Here's how the part is built. I have some questions about the finished solid (model axes, mm). Give positions to 0.01 mm unless a question says otherwise; leave off trailing zeros. Order: outer loops, then holes, each group sorted by start corner. A loop starts at its lowest first (then second) coordinate and runs counter-clockwise, first axis right, second up. Notation, with made-up numbers: M -11.5,68.5 L 44.5,68.5 A27 ccw 44.5,94.5 Z; hole C -22,63.25 d7. An arc over 180 degrees is marked long. One line per item, written item: value. Start each with the question number.
from build123d import *

# Parameters (mm, degrees)
BOSS_EXTRUDE1_DEPTH   = 1
SKETCH8_3_R           = 3
CUT_EXTRUDE1_DEPTH    = 182.285837692
CUT_EXTRUDE2_DEPTH    = 182.285837692
SKETCH10_W            = 14.1
SKETCH10_H            = 14.1
CUT_EXTRUDE3_DEPTH    = 185.637780297
F_3_0MM_DOWEL_HOLE1_D = 3
FILLET1_R             = 1


with BuildPart() as part:
    # Sketch8 → Boss-Extrude1 (new body)
    with BuildSketch(Plane.XY):
        with BuildLine():
            ThreePointArc((116.356165737, 89.593531525), (107.510169126, 99.635128091), (106.844308874, 113.000828513))
            ThreePointArc((106.844308874, 113.000828513), (98.551785503, 130.943955248), (79.67265081, 125.087333856))
            ThreePointArc((79.67265081, 125.087333856), (66.957923375, 111.551078569), (49.923987164, 104.152462611))
            ThreePointArc((49.923987164, 104.152462611), (38.279791522, 92.371702096), (44.581782069, 77.053134095))
            ThreePointArc((44.581782069, 77.053134095), (58.651333394, 69.17496271), (73.852303576, 63.794594289))
            ThreePointArc((73.852303576, 63.794594289), (73.863549821, 63.839319131), (73.875482243, 63.883865813))
            ThreePointArc((73.875482243, 63.883865813), (76.767270103, 63.085390407), (79.729789892, 62.612657392))
            ThreePointArc((79.729789892, 62.612657392), (79.717062502, 62.538833177), (79.702495752, 62.465349771))
            ThreePointArc((79.702495752, 62.465349771), (95.373691885, 60.7573177), (111.111302129, 61.669121188))
            ThreePointArc((111.111302129, 61.669121188), (123.74416397, 73.75113123), (116.356165737, 89.593531525))
        make_face()
        with BuildLine():
            ThreePointArc((109.375963817, 92.019534234), (109.377797318, 92.017499849), (109.379631064, 92.015465685))
            ThreePointArc((109.379631064, 92.015465685), (109.377986421, 92.015505684), (109.376341775, 92.015545509))
            ThreePointArc((109.376341775, 92.015545509), (109.37615287, 92.017539878), (109.375963817, 92.019534234))
        make_face(mode=Mode.SUBTRACT)
        with BuildLine():
            ThreePointArc((56.72077423, 104.000844147), (56.721683918, 104.00117089), (56.7225936, 104.001497652))
            ThreePointArc((56.7225936, 104.001497652), (56.755397532, 103.992206145), (56.788325126, 103.983362865))
            ThreePointArc((56.788325126, 103.983362865), (56.754559843, 103.992142785), (56.72077423, 104.000844147))
        make_face(mode=Mode.SUBTRACT)
        with BuildLine():
            ThreePointArc((103.532400156, 106.396636288), (103.543227812, 106.407709628), (103.554044399, 106.418793781))
            ThreePointArc((103.554044399, 106.418793781), (103.552293137, 106.396310438), (103.550744757, 106.373812212))
            ThreePointArc((103.550744757, 106.373812212), (103.541575551, 106.385226737), (103.532400156, 106.396636288))
        make_face(mode=Mode.SUBTRACT)
        with BuildLine():
            ThreePointArc((104.104138674, 107.788453533), (104.062244422, 107.735361058), (104.021801646, 107.681154775))
            ThreePointArc((104.021801646, 107.681154775), (104.021865069, 107.684582448), (104.021929019, 107.688010111))
            ThreePointArc((104.021929019, 107.688010111), (104.063142491, 107.7381429), (104.104138674, 107.788453533))
        make_face(mode=Mode.SUBTRACT)
    extrude(amount=BOSS_EXTRUDE1_DEPTH)

    # Sketch8_3 → Cut-Extrude1 (cut, through all)
    with BuildSketch(Plane.XY):
        with Locations((106.04559389, 106.21341333)):
            Circle(SKETCH8_3_R)
        with Locations((76.767270103, 63.085390407)):
            Circle(SKETCH8_3_R)
        with Locations((57.420286528, 106.402169345)):
            Circle(SKETCH8_3_R)
    extrude(amount=CUT_EXTRUDE1_DEPTH, mode=Mode.SUBTRACT)

    # Sketch14 → Cut-Extrude2 (cut, through all)
    with BuildSketch(Plane.XY):
        with BuildLine():
            Line((54.297852906, 82.909160119), (55.387130976, 81.231818983))
            ThreePointArc((55.387130976, 81.231818983), (54.003821373, 81.525850516), (54.297852906, 82.909160119))
        make_face()
        with BuildLine():
            Line((56.641344681, 93.934422083), (58.318685817, 95.023700153))
            ThreePointArc((58.318685817, 95.023700153), (56.935376214, 95.317731686), (56.641344681, 93.934422083))
        make_face()
        with BuildLine():
            Line((69.343947781, 92.680208378), (70.433225851, 91.002867242))
            ThreePointArc((70.433225851, 91.002867242), (70.727257384, 92.386176845), (69.343947781, 92.680208378))
        make_face()
        with BuildLine():
            Line((68.089734077, 79.977605278), (66.412392941, 78.888327208))
            ThreePointArc((66.412392941, 78.888327208), (67.795702544, 78.594295675), (68.089734077, 79.977605278))
        make_face()
        with BuildLine():
            Line((75.275056475, 89.973704373), (76.952397611, 91.062982443))
            ThreePointArc((76.952397611, 91.062982443), (75.569088008, 91.357013976), (75.275056475, 89.973704373))
        make_face()
        with BuildLine():
            Line((72.9315647, 78.948442409), (74.02084277, 77.271101273))
            ThreePointArc((74.02084277, 77.271101273), (72.637533167, 77.565132806), (72.9315647, 78.948442409))
        make_face()
        with BuildLine():
            Line((85.046104735, 74.927609498), (86.723445871, 76.016887568))
            ThreePointArc((86.723445871, 76.016887568), (86.429414338, 74.633577965), (85.046104735, 74.927609498))
        make_face()
        with BuildLine():
            Line((89.066937645, 87.042149532), (87.977659575, 88.719490668))
            ThreePointArc((87.977659575, 88.719490668), (89.360969178, 88.425459135), (89.066937645, 87.042149532))
        make_face()
        with BuildLine():
            Line((89.006822445, 93.561321292), (90.684163581, 94.650599362))
            ThreePointArc((90.684163581, 94.650599362), (90.390132048, 93.267289759), (89.006822445, 93.561321292))
        make_face()
        with BuildLine():
            Line((76.89228241, 97.582154203), (77.981560481, 95.904813067))
            ThreePointArc((77.981560481, 95.904813067), (76.598250878, 96.1988446), (76.89228241, 97.582154203))
        make_face()
        with BuildLine():
            Line((91.938377285, 107.353202462), (93.027655356, 105.675861326))
            ThreePointArc((93.027655356, 105.675861326), (93.321686888, 107.059170929), (91.938377285, 107.353202462))
        make_face()
        with BuildLine():
            Line((79.235774185, 108.607416167), (80.913115321, 109.696694237))
            ThreePointArc((80.913115321, 109.696694237), (79.529805718, 109.99072577), (79.235774185, 108.607416167))
        make_face()
        with BuildLine():
            Line((93.908768269, 86.012986663), (95.586109405, 87.102264733))
            ThreePointArc((95.586109405, 87.102264733), (94.202799802, 87.396296266), (93.908768269, 86.012986663))
        make_face()
        with BuildLine():
            Line((91.565276494, 74.987724698), (92.654554564, 73.310383563))
            ThreePointArc((92.654554564, 73.310383563), (91.271244961, 73.604415095), (91.565276494, 74.987724698))
        make_face()
        with BuildLine():
            Line((103.679816529, 70.966891788), (105.357157665, 72.056169858))
            ThreePointArc((105.357157665, 72.056169858), (105.063126132, 70.672860255), (103.679816529, 70.966891788))
        make_face()
        with BuildLine():
            Line((106.611371369, 84.758772958), (107.700649439, 83.081431822))
            ThreePointArc((107.700649439, 83.081431822), (107.994680972, 84.464741425), (106.611371369, 84.758772958))
        make_face()
    extrude(amount=CUT_EXTRUDE2_DEPTH, mode=Mode.SUBTRACT)

    # Sketch10 → Cut-Extrude3 (cut, through all)
    with BuildSketch(Plane(origin=(-22.098060608, 19.345391025, 0), x_dir=(0.9781476007338056, -0.2079116908177598, 0), z_dir=(0, 0, 1))):
        with Locations((68.560828803, 83.69413822)):
            Rectangle(SKETCH10_W, SKETCH10_H)
        with Locations((87.610828803, 83.69413822)):
            Rectangle(SKETCH10_W, SKETCH10_H)
        with Locations((106.660828803, 83.69413822)):
            Rectangle(SKETCH10_W, SKETCH10_H)
        with Locations((87.610828803, 102.74413822)):
            Rectangle(SKETCH10_W, SKETCH10_H)
    extrude(amount=CUT_EXTRUDE3_DEPTH, mode=Mode.SUBTRACT)

    # 3.0mm Dowel Hole1 (through all)
    with Locations(Plane.XY.offset(1)):
        with Locations((70.435309654, 103.157249982)):
            Hole(F_3_0MM_DOWEL_HOLE1_D / 2)

    # Fillet1
    fillet1_edges = [part.edges().sort_by_distance(p)[0] for p in [
        (106.42311517, 103.237261841, 0.5),
        (106.111211206, 109.212695638, 0.5),
        (54.596217873, 105.389926178, 0.5),
        (60.17229201, 107.596516793, 0.5),
        (73.852303576, 63.794594289, 0.5),
        (79.702495752, 62.465349771, 0.5),
    ]]
    fillet(fillet1_edges, radius=FILLET1_R)


solid = part.part
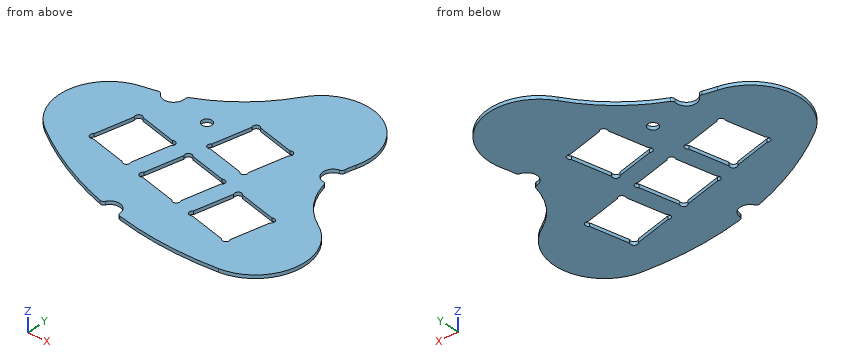
Item 1: I want a section at A-A on x = 82. Write out the boundary of the cut face in (y, z).
Item 2: I want a section at C-C on y = 117. Write out the boundary of the cut face in (x, z).
Item 3: Please list where these lines run through material, in increasing order: probe 1 along Y at (x, z) = (85, 0.95); probe 2 along Y at (x, z) = (95, 0.45); probe 3 along Y at (x, z) = (83, 0.8). Write a range as [from, to].
Item 4: I want a section at D-D on x = 118. Write out the boundary of the cut face in (y, z).
Answer below:
1. outline: M 62.05,0 L 75.58,0 L 75.58,1 L 62.05,1 Z; M 89.99,0 L 95.05,0 L 95.05,1 L 89.99,1 Z; M 109.47,0 L 127.99,0 L 127.99,1 L 109.47,1 Z
2. outline: M 73.36,0 L 107.45,0 L 107.45,1 L 73.36,1 Z
3. probe 1: y = [61.59, 74.94], [89.35, 94.41], [108.83, 130.25]
3. probe 2: y = [60.77, 72.81], [87.53, 132.02]
3. probe 3: y = [61.89, 75.36], [89.78, 94.84], [109.25, 128.88]
4. outline: M 64.52,0 L 88.52,0 L 88.52,1 L 64.52,1 Z
